Verification items for the finished model (mm, model axes). A direction names the side the tool comes from. Round coordinates to 2 decimals unless told otherwise and drop trailing zeros. Write each loop counter-clockwise with the first axis right and the second up, starting at its lowest first coordinate (ties: lowest second). Pieces come first, ordered by that corner, then holes. Notation, with made-up numbers: (-14.5, -9.75) - (35.5, -9.75) arc R18 ccw to (35.5, 4.25) - close; hole circle Ø6 at (78, 13). An arc over 180 degrees is marked (long way). Answer as a JSON object with one key per item and string values. Group by question number.
1) Mould release check, pull along Y, two halves, no side actions. Record for faces 3 (the flat face through (1.229, 0, -1)), 4 (the cylindrical face through (-0.349, -2.657, -0.518)), 5 (the flat face through (0, 0, 5.6)): +Y half, -Y half, draft (parallel to the pull), parting line (faces both ways), or undercut.
2) Thickness scan on line 1 (Z direction, x = -0.8, y = -0.7); line 2 (Y direction, x = 0.4, z = -0.75); line 3 (Z direction, x = -0.55, y = -1.4). Record the ranges inside material, lowest first.
3) Section check B-B (z = 5). Enter the section's corners in (x, y) (3 decimals), then the cut area to 3 significant figures.
4) Set-up check for faces 1 (the flat face through (-0.606, -1.07, -1.41)), 2 (the cylindrical face through (-1.474, 0.065, 2.761)): record each of +Z, -Z, +X, -X, +Y, -Y from which the full face is reachable in a straight line by a thin tool's end or side.
5) Go/stop test with a flat-tipped pin: pin 1 Ø0.7 at (y, z) = (0.5, -1.5) entering from +X. Record where the tip stops, or that it passes through.
```python
from build123d import *

# Parameters (mm, degrees)
CROQUIS1_R              = 1.475
SALIENTE_EXTRUIR1_DEPTH = 5.6
CROQUIS2_R              = 2.68
SALIENTE_EXTRUIR2_DEPTH = 2.15
CORTAR_EXTRUIR1_DEPTH   = 1.5
REDONDEO1_R             = 1.1


with BuildPart() as part:
    # Croquis1 → Saliente-Extruir1 (new body)
    with BuildSketch(Plane.XY):
        Circle(CROQUIS1_R)
    extrude(amount=SALIENTE_EXTRUIR1_DEPTH)

    # Croquis2 → Saliente-Extruir2 (add)
    with BuildSketch(Plane(origin=(0, 0, 0), x_dir=(-1, 0, 0), z_dir=(0, 0, -1))):
        with Locations(Location((0, 0, 0), (0, 0, 180))):
            Circle(CROQUIS2_R)
    extrude(amount=SALIENTE_EXTRUIR2_DEPTH)

    # Croquis3 → Cortar-Extruir1 (cut)
    with BuildSketch(Plane(origin=(0, 0, -2.15), x_dir=(-1, 0, 0), z_dir=(0, 0, -1))):
        Polygon((0, -1.419699202), (1.229495574, -0.709849601), (1.229495574, 0.709849601), (0, 1.419699202), (-1.229495574, 0.709849601), (-1.229495574, -0.709849601), align=None)
    extrude(amount=-CORTAR_EXTRUIR1_DEPTH, mode=Mode.SUBTRACT)

    # Redondeo1
    redondeo1_edges = [part.edges().sort_by_distance(p)[0] for p in [
        (-2.68, 0, -2.15),
    ]]
    fillet(redondeo1_edges, radius=REDONDEO1_R)


solid = part.part
```
Returned:
{
 "1": {"face 3": "undercut", "face 4": "parting line", "face 5": "draft"},
 "2": {"line 1": "-0.65 to 5.6", "line 2": "-2.65 to -1.19, 1.19 to 2.65", "line 3": "-2.15 to 0"},
 "3": {"outline": "circle Ø2.95 at (0, 0)", "area": "6.83 mm2"},
 "4": {"face 1": "-Z", "face 2": "+Z"},
 "5": {"pin 1": "x = 2.65"}
}
